from build123d import *

# Parameters (mm, degrees)
FILLET1_R          = 0.25
FILLET2_R          = 0.3
HEX_2_DEPTH        = 3
SKETCH4_R          = 7.875730731
CUT_EXTRUDE1_DEPTH = 4


with BuildPart() as part:
    # BodySke → Base-Revolve (revolve)
    with BuildSketch(Plane.XY):
        Polygon((0, 0), (0, 5), (6, 5), (6, 3), (15.4455, 3), (16, 2.4455), (16, 0), align=None)
    revolve(axis=Axis((-31.75, 0, 0), (1, 0, 0)))

    # Fillet1
    fillet1_edges = [part.edges().sort_by_distance(p)[0] for p in [
        (6, -3, 0),
    ]]
    fillet(fillet1_edges, radius=FILLET1_R)

    # Fillet2
    fillet2_edges = [part.edges().sort_by_distance(p)[0] for p in [
        (0, -5, 0),
    ]]
    fillet(fillet2_edges, radius=FILLET2_R)

    # Sketch2 → Hex-PreBroach (revolve, cut)
    with BuildSketch(Plane.XY):
        Polygon((0, 2.542), (3, 2.542), (4.467624384, 0), (0, 0), align=None)
    revolve(axis=Axis((0, 0, 0), (1, 0, 0)), mode=Mode.SUBTRACT)

    # Sketch3 → Hex 2 (cut)
    with BuildSketch(Plane(origin=(0, 0, 0), x_dir=(0, 0.5, 0.866025404), z_dir=(-1, 0, 0))):
        Polygon((1.467624384, 2.542), (-1.467624384, 2.542), (-2.935248769, 0), (-1.467624384, -2.542), (1.467624384, -2.542), (2.935248769, 0), align=None)
    extrude(amount=-HEX_2_DEPTH, mode=Mode.SUBTRACT)

    # Sketch4 → Cut-Extrude1 (cut)
    with BuildSketch(Plane(origin=(16, 0, 0), x_dir=(0, 0, -1), z_dir=(1, 0, 0))):
        Circle(SKETCH4_R)
    extrude(amount=-CUT_EXTRUDE1_DEPTH, mode=Mode.SUBTRACT)


solid = part.part
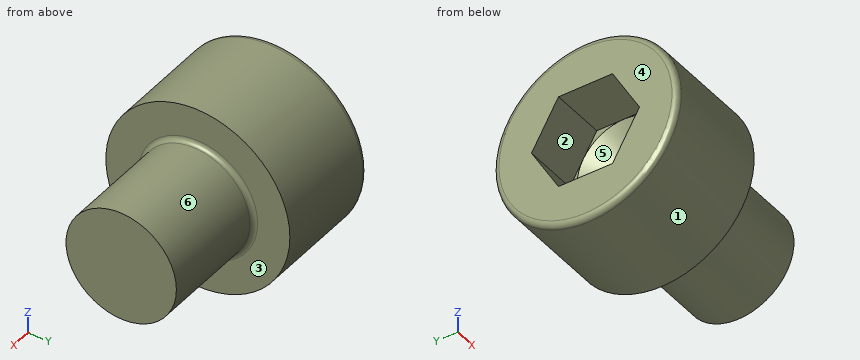
Source: CAD feature listing. Evaluate the final solid. Frame: model axes, mm. Face numbers are marked on the shaded views. A direction names the side the tool comes from. Coordinates: 2 decimals unless noted, no trailing zeros. Loops run counter-clockwise (first coordinate to the right, second up) from the corner with the lowest first, then second, coordinate; pieces in that order, holes last. Notation, with made-up numbers: (84.25, 87.25) - (109.25, 87.25) arc R19 ccw to (109.25, 120.25) - close; hole circle Ø4 at (37, 20). An arc over 180 degrees is marked (long way). One line per question, with ' | ' between items.
1) Section B-B, the plane x = 8.75. Return loops of the section in (y, z).
Report:
outline: circle Ø6 at (0, 0)
2) First-contact query: P1, Ø2, axis at x = 2, z = 2, coming from the +Y side; P2, Ø2, axis at x = 5, y = -4, coming from the -Z side. Flat tips, straight axial feed; report the tip coordinate or a pass-through.
Report:
P1: stops at y = 4.9 | P2: stops at z = -4
3) Section A-A, the plane x = 2.5. Return loops of the section in (y, z), then the cut area to 3 significant figures.
Report:
outline: circle Ø10 at (0, 0); hole (-2.94, 0) - (-1.47, -2.54) - (1.47, -2.54) - (2.94, 0) - (1.47, 2.54) - (-1.47, 2.54) - close | area: 56.2 mm²
4) Section D-D, the plane x = 5. Return loops of the section in (y, z), then the cut area to 3 significant figures.
Report:
outline: circle Ø10 at (0, 0) | area: 78.5 mm²
5) Set-up query: the marked faces 1, 2 and 3. Return all of +Z, -Z, +X, -X, +Y, -Y with unobstructed straight access to the full face (end or side cutting, diameter ignored); none if empty.
Report:
face 1: +X, -X | face 2: -X | face 3: +X
6) Pull-direction query (Z, two-part tool) for the marked faces 4, 5 and 6; classes: released by +Z, released by -Z, zero draft, split by the parting line, or undercut.
Report:
face 4: zero draft | face 5: undercut | face 6: split by the parting line
7) Line query: line 1 along Y through (x, z) = (3.25, -0.25); line 2 along X through (y, z) = (3.5, 1); line 3 along Z through (x, y) = (8.75, 0). Output: solid intervals per line, ascending.
Report:
line 1: y = -4.99 to -2.09, 2.09 to 4.99 | line 2: x = 0 to 6 | line 3: z = -3 to 3
8) Section C-C, the plane x = 3.75. Return loops of the section in (y, z).
Report:
outline: circle Ø10 at (0, 0); hole circle Ø2.49 at (0, 0)
